```python
from build123d import *

# Parameters (mm, degrees)
FILLET_2_R          = 0.05
SKETCH_6_R          = 3.217657182
SKETCH_6_R_2        = 3.1
EXTRUDE_1_DEPTH     = 0.4
FILLET_4_R          = 0.1
CHAMFER_1_SIZE      = 0.1
CHAMFER_1_SIZE2     = 0.076501692
SKETCH_7_R          = 3.5
SKETCH_7_R_2        = 3.35
CUT_EXTRUDE_3_DEPTH = 0.5
CHAMFER_2_SIZE      = 0.01
FILLET_6_R          = 0.1


with BuildPart() as part:
    # 草图2 → 旋转1 (revolve)
    with BuildSketch(Plane.XY, mode=Mode.PRIVATE) as revolve_1_sk:
        Polygon((-0.5, 0), (0, 0), (1.695, 0), (1.695, 0.601670643), (1.446081598, 1.203341286), (0, 1.203341286), align=None)
    revolve(revolve_1_sk.sketch.rotate(Axis((-1.805, 0, 0), (0, 1, 0)), 90), axis=Axis((-1.805, 0, 0), (0, 1, 0)))

    # 圆角2
    fillet_2_edges = [part.edges().sort_by_distance(p)[0] for p in [
        (-1.805, 1.203341286, 1.805),
        (-1.805, 1.203341286, 3.251081598),
    ]]
    fillet(fillet_2_edges, radius=FILLET_2_R)

    # 草图6 → 凸台-拉伸1 (add)
    with BuildSketch(Plane(origin=(0, 1.203341286, 0), x_dir=(1, 0, 0), z_dir=(0, 1, 0))):
        with Locations(Location((-1.805, 0, 0), (0, 0, 270))):
            Circle(SKETCH_6_R)
        with Locations(Location((-1.805, 0, 0), (0, 0, 270))):
            Circle(SKETCH_6_R_2, mode=Mode.SUBTRACT)
    extrude(amount=EXTRUDE_1_DEPTH)

    # 圆角4
    fillet_4_edges = [part.edges().sort_by_distance(p)[0] for p in [
        (-5.022657182, 1.203341286, 0),
        (-1.805, 1.203341286, -3.1),
    ]]
    fillet(fillet_4_edges, radius=FILLET_4_R)

    # 倒角1
    chamfer_1_edges = [part.edges().sort_by_distance(p)[0] for p in [
        (-1.805, 0, 1.305),
    ]]
    chamfer_1_side = [part.faces().sort_by_distance(p)[0] for p in [
        (-1.805, 0, 1.403994949),
    ]]
    chamfer(chamfer_1_edges, length=CHAMFER_1_SIZE, length2=CHAMFER_1_SIZE2, reference=chamfer_1_side[0])

    # 草图7 → 切除-拉伸3 (cut)
    with BuildSketch(Plane(origin=(0, 0.5, 0), x_dir=(1, 0, 0), z_dir=(0, 1, 0))):
        with Locations(Location((-1.805, 0, 0), (0, 0, 90))):
            Circle(SKETCH_7_R)
        with Locations(Location((-1.805, 0, 0), (0, 0, 270))):
            Circle(SKETCH_7_R_2, mode=Mode.SUBTRACT)
    extrude(amount=-CUT_EXTRUDE_3_DEPTH, mode=Mode.SUBTRACT)

    # 倒角2
    chamfer_2_edges = [part.edges().sort_by_distance(p)[0] for p in [
        (-1.805, 0, -3.35),
        (-1.805, 0.5, -3.35),
    ]]
    chamfer(chamfer_2_edges, length=CHAMFER_2_SIZE)

    # 圆角6
    fillet_6_edges = [part.edges().sort_by_distance(p)[0] for p in [
        (-1.805, 0.5, 3.5),
    ]]
    fillet(fillet_6_edges, radius=FILLET_6_R)


solid = part.part
```
Can you work these out from the model? Positions are in its coordinate system, mm. Coordinates: 2 decimals unless noted, no trailing zeros. Loops run counter-clockwise (first coordinate to the right, second up) from the corner with the lowest first, then second, coordinate; pieces in that order, holes last. Notation, with made-up numbers: (84, -34) -> (135, -34) arc R11 cw to (135, -18) -> close; hole circle Ø6 at (15, 89.25). An arc over 180 degrees is marked (long way). Answer as a JSON object with one key per item and string values.
1) Imagine slicing it at A-A (y = 0.2). Please give me the cut outline in (x, z) (3 decimals), then the cut area to 3 significant figures.
Results:
{"outline": "circle Ø6.7 at (-1.805, 0); hole circle Ø2.776 at (-1.805, 0)", "area": "29.2 mm^2"}
2) Thinking about a two-plate mould opening in Z: for faces 1 (the face through (0, 0, 0)), 2 (the face through (-3.84, 0.25, -2.66)), 3 (the face through (0.2, 1.203, 0)), which applies, pulls with the +Z half, pulls with the -Z half, needs draft (parallel to the pull), parting line crosses it, or undercut?
Results:
{"face 1": "needs draft", "face 2": "parting line crosses it", "face 3": "undercut"}
3) If I drill on line 1 (Y direction, x = 0.5, z = -1.75); line 2 (Z direction, x = -1, y = 0.1); line 3 (X direction, y = 0.9, z = -0.25), over which ranges is the centre line in solid material (lowest first)?
Results:
{"line 1": "y = 0 to 1.2", "line 2": "z = -3.25 to -1.08, 1.08 to 3.25", "line 3": "x = -5.17 to -3.47, -0.14 to 1.56"}
